Work out the finished part from the listing and answer in its coordinate system (mm). Face numbers are marked on the shaded views. Coordinates: 2 decimals unless noted, no trailing zeros. Order: outer loops, then holes, each group sorted by start corner. A loop starts at its lowest first (then second) coordinate and runs counter-clockwise, first axis right, second up. Notation, with made-up numbers: M -3,13.25 L 21,13.25 A13 cw 21,33.25 Z; hole C 20,46 d5. An arc over 180 degrees is marked long. Answer in a Markdown table with one row per item. Add a question column.
Item 1: Consider line 1 (Y direction, x = -44, z = 54.5); line 2 (Y direction, x = 43, z = -6); line 3 (X direction, y = 1.25, z = -18). Determine where each line is inside the solid, lowest interval first. Write a range as from..to.
Item 2: The mould has two halves that part along Y. Classify the marked faces 1, 2 and 3: released by +Y, released by -Y, zero draft, split by the parting line, or undercut.
Item 3: The part is cut by section C-C (y = 10.6). Write down the section's boundary in (x, z).
Item 4: The part is cut by section A-A (x = 0). Write down the section's boundary in (y, z), then the cut area to 3 significant figures.
Item 5: The part is cut by section D-D (x = 48). Write down the section's boundary in (y, z), then the cut area to 3 significant figures.
Item 6: Flat-ended cylindrical pins translate along their axes: pin 1 Ø16 at (x, z) = (22.5, 12) entering from +Y; pin 2 Ø7 at (x, y) = (47, 11.5) entering from -Z; pin 3 Ø3 at (x, y) = (-3.5, 1.5) entering from +Z. Find the tip coordinate at first contact, or state that the pin passes through.
Item 7: The part is cut by section B-B (z = 0). Write down the section's boundary in (x, y), then the cut area to 3 significant figures.
Autodesk Inventor part; units mm, degrees
ref_plane "YZ Plane" through (0, 0, 0) normal (1, 0, 0) x (0, 1, 0)
ref_plane "XZ Plane" through (0, 0, 0) normal (0, 1, 0) x (-1, 0, 0)
ref_plane "XY Plane" through (0, 0, 0) normal (0, 0, 1) x (1, 0, 0)
sketch "草圖1" plane through (0, 0, 0) normal (0, 1, 0) x (-1, 0, 0)
  circle A0 centre (0, 0) radius 73
  dimension "d0" = 146
extrude "擠出1" add sketch "草圖1" along normal blind 2.8
sketch "草圖2" plane through (0, 0, 0) normal (0, 0, 1) x (1, 0, 0)
  circle A0 centre (48.9, 10.6) radius 7
  line L0 (73, 0) -> (-73, 0)
  line L1 (73, 0) -> (73, 2.8)
  line L2 (53.4727, 5.3) -> (53.4727, 2.8)
  line L3 (73, 2.8) -> (-73, 2.8)
  line L4 (45.8488, 4.3) -> (45.8488, 2.8)
  point P0 (0, 0)
  point P1 (48.9, 17.6)
  point P2 (41.9, 10.6)
  dimension "d3" = 14
  dimension "d4" = 17.6
  dimension "d5" = 31.1
  dimension "d6" = 1.5
  dimension "d7" = 2.5
extrude "擠出2" add sketch "草圖2" along normal mid plane 58
sketch "草圖3" plane through (0, 2.8, 0) normal (0, 1, 0) x (1, 0, 0)
  line L0 (-41.1, 27.85) -> (45.8488, 27.85)
  line L1 (45.8488, 27.85) -> (45.8488, -27.85)
  line L2 (45.8488, -27.85) -> (-41.1, -27.85)
  line L3 (-41.1, -27.85) -> (-41.1, 27.85)
  line L4 (-38.6, 26.9) -> (45.8488, 26.9)
  line L5 (45.8488, 26.9) -> (45.8488, -26.9)
  line L6 (45.8488, -26.9) -> (-38.6, -26.9)
  line L7 (-38.6, -26.9) -> (-38.6, 26.9)
  line L8 (45.8488, -29) -> (45.8488, 29)
  line L9 (41.9, 29) -> (41.9, -29)
  point P0 (0, 0)
  point P1 (-38.6, 0)
  point P2 (-41.1, 0)
  point P3 (41.9, -27.85)
  point P4 (41.9, -26.9)
  point P5 (41.9, 26.9)
  point P6 (41.9, 27.85)
  dimension "d10" = 55.7
  dimension "d11" = 53.8
  dimension "d12" = 80.5
  dimension "d13" = 83
extrude "擠出3" cut sketch "草圖3" against normal through all contours L0 L9 L4 L7 L6 L2 L3 | L0 L1 L4 L9 | L9 L6 L1 L2
properties part number "平板架"
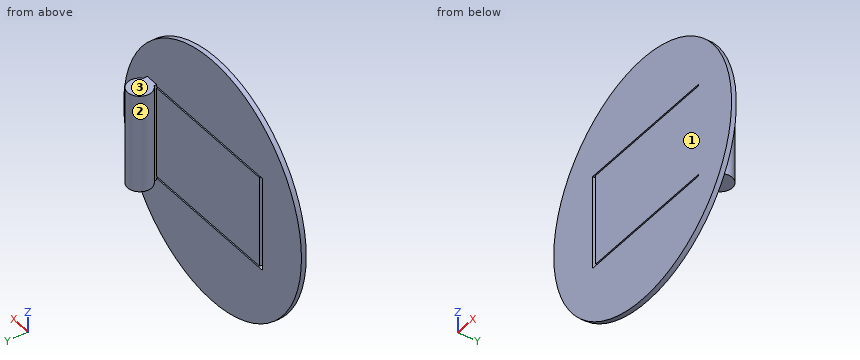
Reply:
| question | item | result |
|---|---|---|
| 1 | line 1 | y = 0..2.8 |
| 1 | line 2 | y = 0..2.8, 6.83..14.37 |
| 1 | line 3 | x = -70.75..-41.1, -38.6..70.75 |
| 2 | face 1 | released by -Y |
| 2 | face 2 | undercut |
| 2 | face 3 | zero draft |
| 3 | outline | M 41.9,-29 L 55.9,-29 L 55.9,29 L 41.9,29 Z |
| 4 | outline | M 0,-73 L 2.8,-73 L 2.8,-27.85 L 0,-27.85 Z; M 0,-26.9 L 2.8,-26.9 L 2.8,26.9 L 0,26.9 Z; M 0,27.85 L 2.8,27.85 L 2.8,73 L 0,73 Z |
| 4 | area | 403 mm2 |
| 5 | outline | M 0,-55 L 2.8,-55 L 2.8,-29 L 17.54,-29 L 17.54,29 L 2.8,29 L 2.8,55 L 0,55 Z |
| 5 | area | 1,160 mm2 |
| 6 | pin 1 | stops at y = 2.8 |
| 6 | pin 2 | stops at z = -29 |
| 6 | pin 3 | stops at z = 72.97 |
| 7 | outline | M -73,0 L -41.1,0 L -41.1,2.8 L -73,2.8 Z; M -38.6,0 L 73,0 L 73,2.8 L 53.47,2.8 L 53.47,5.3 A7 ccw long 45.85,4.3 L 45.85,2.8 L -38.6,2.8 Z |
| 7 | area | 565 mm2 |
